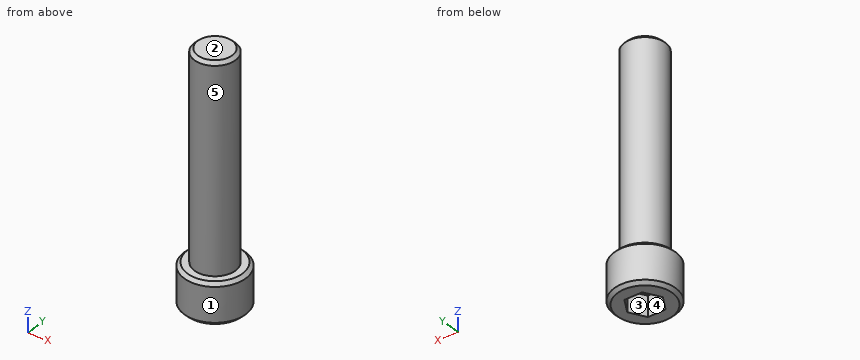
Autodesk Inventor part; units mm, degrees
ref_plane "YZ Plane" through (0, 0, 0) normal (1, 0, 0) x (0, 1, 0)
ref_plane "XZ Plane" through (0, 0, 0) normal (0, 1, 0) x (-1, 0, 0)
ref_plane "XY Plane" through (0, 0, 0) normal (0, 0, 1) x (1, 0, 0)
sketch "Sketch1" plane through (0, 0, 0) normal (0, 0, 1) x (1, 0, 0)
  circle A0 centre (0, 0) radius 3.175
  dimension "d0" = 6.35
extrude "Extrusion1" add sketch "Sketch1" along normal blind 31.75
sketch "Sketch2" plane through (0, 0, 0) normal (0, 0, -1) x (-1, 0, 0)
  circle A0 centre (0, 0) radius 3.175
  circle A1 centre (0, 0) radius 4.7625
  dimension "d3" = 9.525
extrude "Extrusion2" add sketch "Sketch2" along normal blind 6.35 contours A0 | A1
sketch "Sketch3" plane through (0, 0, -6.35) normal (0, 0, -1) x (-1, 0, 0)
  circle A0 centre (0, 0) radius 4.7625
  line L0 (-1.3748, 2.3812) -> (1.3748, 2.3813)
  line L1 (1.3748, 2.3813) -> (2.7496, 0)
  line L2 (2.7496, 0) -> (1.3748, -2.3812)
  line L3 (1.3748, -2.3812) -> (-1.3748, -2.3812)
  line L4 (-1.3748, -2.3812) -> (-2.7496, 0)
  line L5 (-2.7496, 0) -> (-1.3748, 2.3812)
  dimension "d6" = 4.7625
extrude "Extrusion3" cut sketch "Sketch3" against normal blind 3.175 contours L0 L1 L2 L3 L4 L5
chamfer "Chamfer1" distance 0.508 angle 45 3 edges at (-3.175, 0, 31.75) (4.7625, 0, 0) (4.7625, 0, -6.35)
thread "Thread1"
properties part number "14-20 x750" material "Steel"
The model under review builds one solid part; all positions refer to its coordinate system, in mm. Face numbers are marked on the shaded views. A direction names the side the tool comes from. Round coordinates to 2 decimals unless told otherwise and drop trailing zeros. Loops run counter-clockwise (first coordinate to the right, second up) from the corner with the lowest first, then second, coordinate; pieces in that order, holes last. Notation, with made-up numbers: (-33, 86.25) -> (-24, 86.25) arc R11 cw to (-24, 99.25) -> close; hole circle Ø9 at (78.5, 24.5). An arc over 180 degrees is marked (long way). One line per question, with ' | ' between items. Start each with the question number.
Item 1: Draft analysis for pull direction X (two halves, no side actions). For the marked faces 1, 2 and 3, state which applies: +X half, -X half, draft (parallel to the pull), parting line (faces both ways), or undercut.
Item 2: For pin 1 (3 mm diameter, centred on x = 0.5, z = 4, fed in from +Y) (3 decimals); pin 2 (4 mm diameter, centred on x = 3, z = 17, fed in from -Y); pin 3 (1 mm diameter, centred on y = 0, z = 6, fed in from +X) (3 decimals), all flat-tipped, find the tip position at first contact; note any pin that passes through.
Item 3: Machinability: for the marked faces 4 and 5, which of the approach directions +Z, -Z, +X, -X, +Y, -Y give a long, thin tool a straight path to every point of the face, cutting with its end or side? Answer none if there is none.
Item 4: Add section A-A, the plane z = 0.5. Write out the cut boundary in (x, y) (3 decimals), then the cut area to 3 significant figures.
Item 5: Wall thickness on line 1 along Z through (x, y) = (0, 1) (3 decimals); line 2 along Z through (x, y) = (-3.5, -0.25); line 3 along X through (y, z) = (0.25, -4): over which ranges is each line inside the solid? List them lowest first. Write a range as [from, to].
Return value:
1) face 1: parting line | face 2: draft | face 3: undercut
2) pin 1: stops at y = 3.175 | pin 2: stops at y = -3.01 | pin 3: stops at x = 3.175
3) face 4: -Z | face 5: +Z
4) outline: circle Ø6.35 at (0, 0) | area: 31.7 mm2
5) line 1: z = [-3.175, 31.75] | line 2: z = [-6.35, 0] | line 3: x = [-4.76, -2.61], [2.61, 4.76]
